The model under review builds one solid part; all positions refer to its coordinate system, in mm. A direction names the side the tool comes from. Coordinates: 2 decimals unless noted, no trailing zeros. Order: outer loops, then holes, each group sorted by start corner. A loop starts at its lowest first (then second) coordinate and runs counter-clockwise, first axis right, second up. Notation, with made-up numbers: M 11.5,-25 L 39.5,-25 A30 ccw 39.5,14 Z; hole C 48,-6.5 d8. An arc over 180 degrees is marked long. One line per item, written item: value.
```python
from build123d import *

# Parameters (mm, degrees)
SKETCH1_W           = 127
SKETCH1_H           = 76.2
BOSS_EXTRUDE1_DEPTH = 12.7
SKETCH2_W           = 12.7
SKETCH2_H           = 76.2
BOSS_EXTRUDE2_DEPTH = 38.1
FILLET1_R           = 12.7
FILLET2_R           = 12.7
BOSS_EXTRUDE3_REACH = 142.563
SKETCH7_R           = 9.525
SKETCH5_R           = 6.35
CUT_EXTRUDE1_DEPTH  = 38.1
SKETCH8_R           = 6.35
CUT_EXTRUDE2_DEPTH  = 38.1


with BuildPart() as part:
    # Sketch1 → Boss-Extrude1 (new body)
    with BuildSketch(Plane(origin=(0, 0, 0), x_dir=(1, 0, 0), z_dir=(0, 1, 0))):
        with Locations((63.5, 38.1)):
            Rectangle(SKETCH1_W, SKETCH1_H)
    extrude(amount=BOSS_EXTRUDE1_DEPTH)

    # Sketch2 → Boss-Extrude2 (add)
    with BuildSketch(Plane(origin=(0, 12.7, 0), x_dir=(1, 0, 0), z_dir=(0, 1, 0))):
        with Locations((120.65, 38.1)):
            Rectangle(SKETCH2_W, SKETCH2_H)
    extrude(amount=-BOSS_EXTRUDE2_DEPTH)

    # Fillet1
    fillet1_edges = [part.edges().sort_by_distance(p)[0] for p in [
        (120.65, -25.4, 0),
    ]]
    fillet(fillet1_edges, radius=FILLET1_R)

    # Fillet2
    fillet2_edges = [part.edges().sort_by_distance(p)[0] for p in [
        (120.65, -25.4, -76.2),
    ]]
    fillet(fillet2_edges, radius=FILLET2_R)

    # Boss-Extrude3: up to this face of the body (flat: up to its plane)
    boss_extrude3_end = Plane(part.part.faces().sort_by_distance((63.5, 12.7, -38.1))[0])
    # Sketch7 → Boss-Extrude3 (add, up to the picked face)
    with BuildSketch(Plane(origin=(69.85, 69.85, 0), x_dir=(0, 0, -1), z_dir=(0.7071067811865488, 0.7071067811865464, 0)), mode=Mode.PRIVATE) as boss_extrude3_sk1:
        with BuildLine():
            Line((63.678120433, -80.82230509), (12.878120433, -80.82230509))
            Line((12.878120433, -80.82230509), (12.878120433, -30.02230509))
            ThreePointArc((12.878120433, -30.02230509), (38.278120433, -4.62230509), (63.678120433, -30.02230509))
            Line((63.678120433, -30.02230509), (63.678120433, -80.82230509))
        make_face()
        with Locations(Location((38.278120433, -30.02230509, 0), (0, 0, 90))):
            Circle(SKETCH7_R, mode=Mode.SUBTRACT)
    boss_extrude3_tool1 = split(extrude(boss_extrude3_sk1.sketch, amount=-BOSS_EXTRUDE3_REACH, mode=Mode.PRIVATE), bisect_by=boss_extrude3_end, keep=Keep.BOTH, mode=Mode.PRIVATE)
    add(boss_extrude3_tool1.solids().sort_by(Axis((102.751477, 36.948523, -38.27812), (-0.7071067811865488, -0.7071067811865464, 0)))[0])

    # Sketch5 → Cut-Extrude1 (cut)
    with BuildSketch(Plane(origin=(0, 12.7, 0), x_dir=(1, 0, 0), z_dir=(0, 1, 0))):
        with Locations(Location((12.7, 63.5, 0), (0, 0, 270))):
            Circle(SKETCH5_R)
        with Locations(Location((12.7, 12.7, 0), (0, 0, 270))):
            Circle(SKETCH5_R)
    extrude(amount=-CUT_EXTRUDE1_DEPTH, mode=Mode.SUBTRACT)

    # Sketch8 → Cut-Extrude2 (cut)
    with BuildSketch(Plane(origin=(127, 0, 0), x_dir=(0, 0, -1), z_dir=(1, 0, 0))):
        with Locations((12.7, -12.7)):
            Circle(SKETCH8_R)
        with Locations((63.5, -12.7)):
            Circle(SKETCH8_R)
    extrude(amount=-CUT_EXTRUDE2_DEPTH, mode=Mode.SUBTRACT)


solid = part.part
```
(1) Tool access review of faces 4 (the flat face through (48, 12.7, -64)), 5 (the flat face through (91, 21, -63.678)), 6 (the flat face through (56, 0, -39)): name each direction out of +Z, -Z, +X, -X, +Y, -Y from which nothing blocks a thin tool from reaching the whole face with its end or side.
Geometry results:
face 4: -X, +Y
face 5: -Z, +X, -X, +Y
face 6: +Z, -Z, -X, -Y
(2) We need section B-B, the plane z = -61. State the section outline as (x, y) points, plus the area to 3 significant figures.
Geometry results:
outline: M 0,0 L 6.86,0 L 6.86,12.7 L 0,12.7 Z; M 18.54,0 L 114.3,0 L 114.3,-6.86 L 127,-6.86 L 127,12.7 L 83.05,56.65 L 39.1,12.7 L 18.54,12.7 Z; M 114.3,-25.4 L 127,-25.4 L 127,-18.54 L 114.3,-18.54 Z
area: 3,570 mm2
(3) We need section D-D, the plane x = 101.5. State the section outline as (y, z) points, plus the area to 3 significant figures.
Geometry results:
outline: M 0,-76.2 L 12.7,-76.2 L 12.7,-63.68 L 38.2,-63.68 L 38.2,-12.88 L 12.7,-12.88 L 12.7,0 L 0,0 Z
area: 2,260 mm2
(4) We need section C-C, the plane y = 2.5. State the section outline as (x, z) points.
Geometry results:
outline: M 0,-76.2 L 127,-76.2 L 127,0 L 0,0 Z; hole C 12.7,-63.5 d12.7; hole C 12.7,-12.7 d12.7
(5) We need section A-A, the plane x = 12.7. State the section outline as (y, z) points.
Geometry results:
outline: M 0,-76.2 L 12.7,-76.2 L 12.7,-69.85 L 0,-69.85 Z; M 0,-57.15 L 12.7,-57.15 L 12.7,-19.05 L 0,-19.05 Z; M 0,-6.35 L 12.7,-6.35 L 12.7,0 L 0,0 Z
(6) Mouldability with a two-part tool opening along Y and no side actions: class faces 1 (the flat face through (99.7, 40, -38.6)), 2 (the cylindrical face through (120.74, -21.58, -3.62)), 3 (the flat face through (55, 12.7, -38)) as +Y half, -Y half, draft (parallel to the pull), parting line (faces both ways), or undercut.
Geometry results:
face 1: +Y half
face 2: -Y half
face 3: undercut
(7) For L1, parallel to Z at x = 117, y = -12; L2, parallel to X at y = 4, z = -63.5; L3, parallel to X at y = -13.5, z = -56, list the stretches that pass through material, from the lowest coordinate up.
Geometry results:
L1: z = -76.2 to -69.81, -57.19 to -19.01, -6.39 to 0
L2: x = 0 to 6.35, 19.05 to 127
L3: x = 114.3 to 127
(8) Insertion check: pin 1 Ø14.5 at (y, z) = (-12.7, -12.7) entering from -X; pin 2 Ø4 at (x, z) = (102.5, -26) entering from +Y; pin 3 Ø18 at (x, y) = (77, 27) entering from -Z. Each pin has a flat end and moves straight along its axis. Give the tip position at first contact, or say it passes through.
Geometry results:
pin 1: stops at x = 114.3
pin 2: stops at y = 39.2
pin 3: stops at z = -63.68
